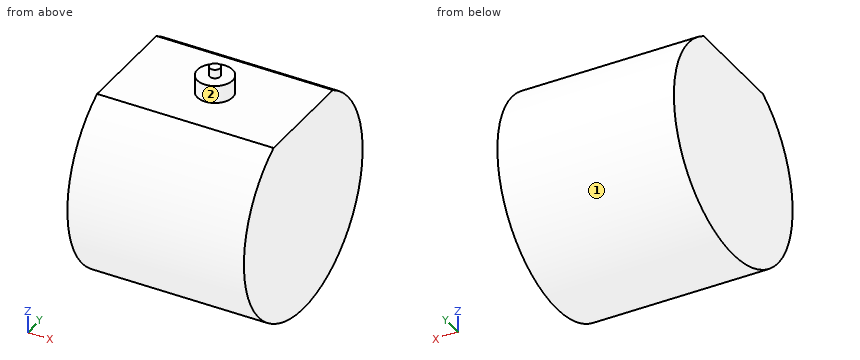
from build123d import *

# Parameters (mm, degrees)
F1_DEPTH = 127
F2_R     = 12.7
F3_DEPTH = 12.7
F4_R     = 3.81
F5_DEPTH = 6.35


with BuildPart() as f1:
    # F0 (on Right) → F1 (new body)
    with BuildSketch(Plane.YZ):
        with BuildLine():
            Line((16.657175, 68.595961), (-59.542825, 68.595961))
            ThreePointArc((-59.542825, 68.595961), (-21.442825, -73.595175), (16.657175, 68.595961))
        make_face()
    extrude(amount=F1_DEPTH)

    # F2 (on face) → F3 (join)
    with BuildSketch(Plane.XY.offset(68.595961)):
        with Locations((63.5, -21.442825)):
            Circle(F2_R)
    extrude(amount=F3_DEPTH)

    # F4 (on face) → F5 (join)
    with BuildSketch(Plane.XY.offset(81.295961)):
        with Locations((63.5, -21.442825)):
            Circle(F4_R)
    extrude(amount=F5_DEPTH)


solid = f1.part
For this review, take the finished solid that the model builds, in its own axes (mm). Face numbers are marked on the shaded views. A direction names the side the tool comes from. Give positions to 0.01 mm unless a question says otherwise; leave off trailing zeros. Loops run counter-clockwise (first coordinate to the right, second up) from the corner with the lowest first, then second, coordinate; pieces in that order, holes last. Notation, with made-up numbers: M 66.25,-27 L 113.25,-27 A12 cw 113.25,-18 Z; hole C 0,38.25 d8. An arc over 180 degrees is marked long. Put each result on its own line as item: value. Start each with the question number.
(1) Add section C-C, the plane z = -47. Write out the cut boundary in (x, y).
(2) Add section D-D, the plane x = 11. Write out the cut boundary in (y, z), then the cut area to 3 significant figures.
(3) Wall thickness on L1, parallel to Z at x = 18, y = -19.5; L2, parallel to Z at x = 43.5, y = 39; L3, parallel to Y at x = 44, z = 53: over which ranges is each line inside the solid? List them lowest first.
(4) For pin 1 (3 mm diameter, centred on x = 103.5, y = 25.5, fed in from +Z); pin 2 (4 mm diameter, centred on x = 85, y = -71.5, fed in from +Z); pin 3 (6 mm diameter, centred on x = 72.5, z = -5.5, fed in from -Y), all flat-tipped, find the tip position at first contact; note any pin that passes through.
(5) Add section A-A, the plane x = 63.5. Write out the cut boundary in (y, z).
(6) Machinability: for the marked faces 1 and 2, which of the approach directions +Z, -Z, +X, -X, +Y, -Y give a long, thin tool a straight path to every point of the face, cutting with its end or side? Answer none if there is none.
(7) Add section B-B, the plane y = -70. Write out the cut boundary in (x, z).
Result:
1. outline: M 0,-79.29 L 127,-79.29 L 127,36.4 L 0,36.4 Z
2. outline: M -59.54,68.6 A76.2 ccw long 16.66,68.6 Z
2. area: 17,700 mm^2
3. L1: z = -73.57 to 68.6
3. L2: z = -43.8 to 49.01
3. L3: y = -78.6 to 35.71
4. pin 1: stops at z = 63.77
4. pin 2: stops at z = 61.74
4. pin 3: stops at y = -97.47
5. outline: M -59.54,68.6 A76.2 ccw long 16.66,68.6 L -8.74,68.6 L -8.74,81.3 L -17.63,81.3 L -17.63,87.65 L -25.25,87.65 L -25.25,81.3 L -34.14,81.3 L -34.14,68.6 Z
6. face 1: +X, -X
6. face 2: +Z
7. outline: M 0,-56.12 L 127,-56.12 L 127,61.33 L 0,61.33 Z
